```python
from build123d import *

# Parameters (mm, degrees)
BOSS_EXTRUDE1_DEPTH = 4
SKETCH2_W           = 5
SKETCH2_H           = 1.6
BOSS_EXTRUDE2_DEPTH = 4
SKETCH5_R           = 1.45
CUT_EXTRUDE3_DEPTH  = 14.2
SKETCH7_R           = 2.375
CUT_EXTRUDE6_DEPTH  = 15
SKETCH8_R           = 2.094517613
BOSS_EXTRUDE3_DEPTH = 1
BOSS_EXTRUDE4_DEPTH = 3


with BuildPart() as part:
    # Sketch1 → Boss-Extrude1 (new body)
    with BuildSketch(Plane.XY):
        with BuildLine():
            Line((-9.975, 0), (9.975, 0))
            Line((9.975, 0), (9.975, 10))
            Line((9.975, 10), (9.128095747, 20.764013839))
            Line((9.128095747, 20.764013839), (4.125144755, 22.256540984))
            Line((4.125144755, 22.256540984), (3.110466203, 15.675))
            ThreePointArc((3.110466203, 15.675), (0, 11.175), (-3.110466203, 15.675))
            Line((-3.110466203, 15.675), (-4.125144755, 22.256540984))
            Line((-4.125144755, 22.256540984), (-9.128095747, 20.764013839))
            Line((-9.128095747, 20.764013839), (-9.975, 10))
            Line((-9.975, 10), (-9.975, 0))
        make_face()
    extrude(amount=BOSS_EXTRUDE1_DEPTH)

    # Sketch2 → Boss-Extrude2 (add)
    with BuildSketch(Plane(origin=(0, 0, 0), x_dir=(-1, 0, 0), z_dir=(0, 0, -1))):
        with Locations((0, -0.8)):
            Rectangle(SKETCH2_W, SKETCH2_H)
    extrude(amount=-BOSS_EXTRUDE2_DEPTH)

    # Sketch5 → Cut-Extrude3 (cut)
    with BuildSketch(Plane.XY.offset(4)):
        with Locations((6.975, 5)):
            Circle(SKETCH5_R)
    cut_extrude3 = extrude(amount=-CUT_EXTRUDE3_DEPTH, mode=Mode.SUBTRACT)

    # Mirror1: Cut-Extrude3 across plane
    add(cut_extrude3.mirror(Plane(origin=(0, 0, 0), x_dir=(0, 0, 1), z_dir=(1, 0, 0))), mode=Mode.SUBTRACT)

    # Sketch7 → Cut-Extrude6 (cut)
    with BuildSketch(Plane.XY.offset(4)):
        with Locations((0, 5.1)):
            Circle(SKETCH7_R)
    extrude(amount=-CUT_EXTRUDE6_DEPTH, mode=Mode.SUBTRACT)

    # Sketch8 → Boss-Extrude3 (add)
    with BuildSketch(Plane.XY.offset(4)):
        with Locations((5.849630313, 14.875934422)):
            Circle(SKETCH8_R)
        with Locations(Location((-5.849630313, 14.875934422, 0), (0, 0, 180))):
            Circle(SKETCH8_R)
    extrude(amount=BOSS_EXTRUDE3_DEPTH)

    # Sketch9 → Boss-Extrude4 (add)
    with BuildSketch(Plane.XY.offset(4)):
        Polygon((4.125144755, 22.256540984), (3.606658762, 18.893469192), (9.406048413, 17.23128114), (9.128095747, 20.764013839), align=None)
        Polygon((-9.128095747, 20.764013839), (-4.125144755, 22.256540984), (-3.606658762, 18.893469192), (-9.406048413, 17.23128114), align=None)
    extrude(amount=BOSS_EXTRUDE4_DEPTH)


solid = part.part
```
For this review, take the finished solid that the model builds, in its own axes (mm). A direction names the side the tool comes from. Coordinates: 2 decimals unless noted, no trailing zeros. Write each loop counter-clockwise with the first axis right and the second up, starting at its lowest first coordinate (ties: lowest second). Pieces come first, ordered by that corner, then holes. Notation, with made-up numbers: (23, -9) - (28, -9) arc R18 cw to (28, 17) - close; hole circle Ø4 at (36, 47.25). An arc over 180 degrees is marked (long way). Answer in a Markdown table with one row per item. Add a question column.
Q1. For probe 1 along Y at (x, z) = (0, 2) (3 decimals); probe 2 along X at (y, z) = (16, 4.75); probe 3 along X at (y, z) = (4.5, 1.75) (3 decimals), list the stretches that pass through material, from the lowest coordinate up.
Q2. We need section B-B, the plane z = 6.25. State the section outline as (x, y) points, and give its area (3 significant figures).
Q3. For P1, Ø6, axis at x = -0.5, y = 5.5, coming from the +Z side; P2, Ø0.5, axis at y = -1, z = 1.5, coming from the +X side; P3, Ø2, axis at x = 5.5, y = 15.5, coming from the +Z side, all flat-tipped, find the tip position at first contact; note any pin that passes through.
Q4. Draft analysis for pull direction Y (two halves, no side actions). For faces 4 (the flat face through (6.66, 21.5, 3.45)), 5 (the flat face through (-6, 0, 2)), 6 (the flat face through (0, 10, 0)), 7 (the cylindrical face through (-0.51, 2.78, 2.03)), state which applies: +Y half, -Y half, draft (parallel to the pull), parting line (faces both ways), or undercut.
Q5. We need section A-A, the plane x = 0. State the section outline as (y, z) points (3 decimals).
Q6. We need section C-C, the plane y = 14.5. State the section outline as (x, z) points (3 decimals).
Q7. Tool access review of faces 1 (the flat face through (6, 15, 5)), 2 (the flat face through (6, 0, 2)), 3 (the cylindrical face through (-5.58, 12.8, 4.49)): name each direction out of +Z, -Z, +X, -X, +Y, -Y from which nothing blocks a thin tool from reaching the whole face with its end or side.
Q8. We need section D-D, the plane z = 2.5. State the section outline as (x, y) points (3 decimals), and give its area (3 significant figures).
Answer list:
| question | item | result |
|---|---|---|
| 1 | probe 1 | y = -1.6 to 2.725, 7.475 to 11.175 |
| 1 | probe 2 | x = -7.62 to -4.08, 4.08 to 7.62 |
| 1 | probe 3 | x = -9.975 to -8.336, -5.614 to -2.298, 2.298 to 5.614, 8.336 to 9.975 |
| 2 | outline | (-9.41, 17.23) - (-3.61, 18.89) - (-4.13, 22.26) - (-9.13, 20.76) - close; (3.61, 18.89) - (9.41, 17.23) - (9.13, 20.76) - (4.13, 22.26) - close |
| 2 | area | 37.6 mm2 |
| 3 | P1 | stops at z = 4 |
| 3 | P2 | stops at x = 2.5 |
| 3 | P3 | stops at z = 5 |
| 4 | face 4 | +Y half |
| 4 | face 5 | -Y half |
| 4 | face 6 | draft |
| 4 | face 7 | undercut |
| 5 | outline | (-1.6, 0) - (2.725, 0) - (2.725, 4) - (-1.6, 4) - close; (7.475, 0) - (11.175, 0) - (11.175, 4) - (7.475, 4) - close |
| 6 | outline | (-9.621, 0) - (-3.325, 0) - (-3.325, 4) - (-3.789, 4) - (-3.789, 5) - (-7.91, 5) - (-7.91, 4) - (-9.621, 4) - close; (3.325, 0) - (9.621, 0) - (9.621, 4) - (7.91, 4) - (7.91, 5) - (3.789, 5) - (3.789, 4) - (3.325, 4) - close |
| 7 | face 1 | +Z, +X, -X, -Y |
| 7 | face 2 | +Z, -Z, +X, -Y |
| 7 | face 3 | +Z |
| 8 | outline | (-9.975, 0) - (-2.5, 0) - (-2.5, -1.6) - (2.5, -1.6) - (2.5, 0) - (9.975, 0) - (9.975, 10) - (9.128, 20.764) - (4.125, 22.257) - (3.11, 15.675) arc R3.325 cw (long way) to (-3.11, 15.675) - (-4.125, 22.257) - (-9.128, 20.764) - (-9.975, 10) - close; hole circle Ø2.9 at (-6.975, 5); hole circle Ø4.75 at (0, 5.1); hole circle Ø2.9 at (6.975, 5) |
| 8 | area | 329 mm2 |
